from build123d import *

# Parameters (mm, degrees)
SKETCH_1_R      = 1.05
SKETCH_1_R_2    = 1.585
SKETCH_1_W      = 9
SKETCH_1_H      = 9
SKETCH_1_W_2    = 11
SKETCH_1_H_2    = 12
SKETCH_1_R_3    = 4
EXTRUDE_1_DEPTH = 2


with BuildPart() as part:
    # 草图1 → 凸台-拉伸1 (new body)
    with BuildSketch(Plane(origin=(0, 0, 0), x_dir=(1, 0, 0), z_dir=(0, 1, 0))):
        Polygon((70.16, 0), (0, 0), (0, -115), (99.16, -115), (99.16, -101), (94.16, -101), (94.16, -13), (99.16, -13), (99.16, 0), (88.16, 0), (88.16, -32), (70.16, -32), align=None)
        with Locations(Location((15.69, -113, 0), (0, 0, 270))):
            Circle(SKETCH_1_R, mode=Mode.SUBTRACT)
        with Locations(Location((22.16, -87.2, 0), (0, 0, 270))):
            Circle(SKETCH_1_R_2, mode=Mode.SUBTRACT)
        Polygon((43.16, -48.5), (43.16, -42), (57.16, -42), (57.16, -49), (56.5, -49), (56.5, -73), (32, -73), (32, -48.5), align=None, mode=Mode.SUBTRACT)
        with Locations(Location((65.96, -95, 0), (0, 0, 270))):
            Circle(SKETCH_1_R, mode=Mode.SUBTRACT)
        with Locations(Location((66.66, -87.2, 0), (0, 0, 270))):
            Circle(SKETCH_1_R_2, mode=Mode.SUBTRACT)
        with Locations(Location((78.69, -113, 0), (0, 0, 270))):
            Circle(SKETCH_1_R, mode=Mode.SUBTRACT)
        with Locations(Location((90.66, -101.2, 0), (0, 0, 270))):
            Circle(SKETCH_1_R_2, mode=Mode.SUBTRACT)
        with Locations(Location((91.36, -95, 0), (0, 0, 270))):
            Circle(SKETCH_1_R, mode=Mode.SUBTRACT)
        Polygon((50.16, -83.5), (50.16, -77.5), (54.66, -77.5), (54.66, -83), (63.16, -83), (63.16, -93), (53.16, -93), (53.16, -83.5), align=None, mode=Mode.SUBTRACT)
        with Locations((78.66, -67.5)):
            Rectangle(SKETCH_1_W, SKETCH_1_H, mode=Mode.SUBTRACT)
        with Locations(Location((22.16, -27.46, 0), (0, 0, 270))):
            Circle(SKETCH_1_R_2, mode=Mode.SUBTRACT)
        with Locations((19.5, -15)):
            Rectangle(SKETCH_1_W_2, SKETCH_1_H_2, mode=Mode.SUBTRACT)
        with Locations(Location((15.69, -2, 0), (0, 0, 270))):
            Circle(SKETCH_1_R, mode=Mode.SUBTRACT)
        with Locations(Location((65.96, -54, 0), (0, 0, 270))):
            Circle(SKETCH_1_R, mode=Mode.SUBTRACT)
        with Locations(Location((56.66, -33.5, 0), (0, 0, 270))):
            Circle(SKETCH_1_R_3, mode=Mode.SUBTRACT)
        with Locations(Location((91.36, -54, 0), (0, 0, 270))):
            Circle(SKETCH_1_R, mode=Mode.SUBTRACT)
        with Locations(Location((66.66, -27.46, 0), (0, 0, 270))):
            Circle(SKETCH_1_R_2, mode=Mode.SUBTRACT)
        with Locations(Location((90.66, -13.2, 0), (0, 0, 270))):
            Circle(SKETCH_1_R_2, mode=Mode.SUBTRACT)
        with Locations(Location((8.12, -12.2, 0), (0, 0, 270))):
            Circle(SKETCH_1_R_2, mode=Mode.SUBTRACT)
        with Locations(Location((8.62, -38.06, 0), (0, 0, 270))):
            Circle(SKETCH_1_R_2, mode=Mode.SUBTRACT)
    extrude(amount=EXTRUDE_1_DEPTH)


solid = part.part
The model under review builds one solid part; all positions refer to its coordinate system, in mm. Give positions to 0.01 mm unless a question says otherwise; leave off trailing zeros. Write each loop counter-clockwise with the first axis right and the second up, starting at its lowest first coordinate (ties: lowest second). Pieces come first, ordered by that corner, then holes.
1. Add section D-D, the plane y = 0.5. Count the separate pieces of the cut face and the enclosed holes in it, plus the area to 3 significant figures.
2. Add section A-A, the plane z = 33.5. Write out the cut boundary in (x, y), plus the area to 3 significant figures.
3. For P1, Ø0.6, axis at y = 1, z = 80.5, coming from the +X side; P2, Ø1, axis at x = 78.5, y = 1, coming from the -Z side, all flat-tipped, find the tip position at first contact; note any pin that passes through.
4. Add section C-C, the plane x = 22.16. Write out the cut boundary in (y, z) (3 decimals), plus the area to 3 significant figures.
5. Add section B-B, the plane x = 36.5. Write out the cut boundary in (y, z).
6. Wall thickness on L1, parallel to Z at x = 78.69, y = 1; L2, parallel to X at y = 0.4, z = 95; L3, parallel to X at y = 0.6, z = 15: over which ranges is each line inside the solid? List them lowest first.
7. Draft analysis for pull direction X (two halves, no side actions). For faces 1 (the flat face through (60, 2, 57)), 2 (the cylindrical face through (21.2, 0.99, 85.94)), state which applies: +X half, -X half, draft (parallel to the pull), parting line (faces both ways), or undercut.
Worked answers:
1. separate pieces: 1
1. enclosed holes: 20
1. area: 9,220 mm2
2. outline: (0, 0) - (52.66, 0) - (52.66, 2) - (0, 2) - close; (60.66, 0) - (94.16, 0) - (94.16, 2) - (60.66, 2) - close
2. area: 172 mm2
3. P1: stops at x = 94.16
3. P2: stops at z = 32
4. outline: (0, 0) - (2, 0) - (2, 9) - (0, 9) - close; (0, 21) - (2, 21) - (2, 25.875) - (0, 25.875) - close; (0, 29.045) - (2, 29.045) - (2, 85.615) - (0, 85.615) - close; (0, 88.785) - (2, 88.785) - (2, 115) - (0, 115) - close
4. area: 193 mm2
5. outline: (0, 0) - (2, 0) - (2, 48.5) - (0, 48.5) - close; (0, 73) - (2, 73) - (2, 115) - (0, 115) - close
6. L1: z = 32 to 63, 72 to 111.95, 114.05 to 115
6. L2: x = 0 to 64.91, 67.01 to 90.31, 92.41 to 94.16
6. L3: x = 0 to 14, 25 to 70.16, 88.16 to 94.16
7. face 1: draft
7. face 2: undercut
